Could you check a few things on this model? Use its own coordinates, in mm. Coordinates: 2 decimals unless noted, no trailing zeros. Loops run counter-clockwise (first coordinate to the right, second up) from the corner with the lowest first, then second, coordinate; pieces in that order, holes last. Notation, with made-up numbers: (61.5, 26.25) - (87.5, 26.25) arc R31 ccw to (87.5, 55.25) - close; hole circle Ø10 at (46, 24.25). An arc over 180 degrees is marked (long way). Put each result on its own line as item: value. Start each with the question number.
```python
from build123d import *

# Parameters (mm, degrees)
SKETCH1_W           = 50
SKETCH1_H           = 60
SKETCH1_R           = 4
BOSS_EXTRUDE1_DEPTH = 3
SKETCH2_R           = 5.25
CUT_EXTRUDE2_DEPTH  = 40.166312055


with BuildPart() as part:
    # Sketch1 → Boss-Extrude1 (new body)
    with BuildSketch(Plane.XY):
        Rectangle(SKETCH1_W, SKETCH1_H)
        with Locations((-10, 19)):
            Circle(SKETCH1_R, mode=Mode.SUBTRACT)
    extrude(amount=BOSS_EXTRUDE1_DEPTH)

    # Sketch2 → Cut-Extrude2 (cut, through all)
    with BuildSketch(Plane.XY):
        with Locations((13, 19)):
            Circle(SKETCH2_R)
    extrude(amount=CUT_EXTRUDE2_DEPTH, mode=Mode.SUBTRACT)


solid = part.part
```
(1) I need wall thicknesses on L1, parallel to Y at x = -10, z = 1.1; L2, parallel to Y at x = 13, z = 1.8; L3, parallel to X at y = 22.5, z = 0.5. Which ranges of each line are inside material? Lowest first, please. Write a range as [from, to].
(2) I want a section at D-D on x = -10. List the corners of the cut face in (y, z) for me.
(3) If we mould it in two halves opening along Y, with no side actions, what happens to faces 1 (the cylindrical face through (-10.521, 22.966, 1.479)), 2 (the flat face through (0, 0, 0)), 3 (the flat face through (0, 30, 1)), 4 (the cylindrical face through (8.83, 15.81, 1.48))? For each: pulls with the +Y half, pulls with the -Y half, needs draft (parallel to the pull), parting line crosses it, or undercut.
(4) I want a section at B-B on x = 13. List the corners of the cut face in (y, z) for me, and give its area (4 significant figures).
(5) I want a section at C-C on z = 1.95. List the corners of the cut face in (x, y) for me, and give its area (3 significant figures).
(6) For pin 1 Ø17 at (x, y) = (13, 19) entering from +Z; pin 2 Ø6.5 at (x, y) = (-10, 19) entering from -Z, each with a flat end and sliding along its axis, tell me the tip position at first contact or that it passes through.
(7) I want a section at A-A on y = 19. List the corners of the cut face in (x, z) for me.
Answer sheet:
1. L1: y = [-30, 15], [23, 30]
1. L2: y = [-30, 13.75], [24.25, 30]
1. L3: x = [-25, -11.94], [-8.06, 9.09], [16.91, 25]
2. outline: (-30, 0) - (15, 0) - (15, 3) - (-30, 3) - close; (23, 0) - (30, 0) - (30, 3) - (23, 3) - close
3. face 1: undercut
3. face 2: needs draft
3. face 3: pulls with the +Y half
3. face 4: undercut
4. outline: (-30, 0) - (13.75, 0) - (13.75, 3) - (-30, 3) - close; (24.25, 0) - (30, 0) - (30, 3) - (24.25, 3) - close
4. area: 148.5 mm^2
5. outline: (-25, -30) - (25, -30) - (25, 30) - (-25, 30) - close; hole circle Ø8 at (-10, 19); hole circle Ø10.5 at (13, 19)
5. area: 2,860 mm^2
6. pin 1: stops at z = 3
6. pin 2: passes through
7. outline: (-25, 0) - (-14, 0) - (-14, 3) - (-25, 3) - close; (-6, 0) - (7.75, 0) - (7.75, 3) - (-6, 3) - close; (18.25, 0) - (25, 0) - (25, 3) - (18.25, 3) - close
